from build123d import *

# Parameters (mm, degrees)
EXTRUDE_START                 = -32
EXTRUDE_15_DEPTH              = 64
CUT_EXTRUDE_1_DEPTH           = 100
CUT_EXTRUDE_1_DEPTH_BACK      = 100
SKETCH_2_R                    = 3.2
CUT_EXTRUDE_1_2_DEPTH         = 100
CUT_EXTRUDE_1_2_DEPTH_BACK    = 100
SKETCH_3_R                    = 3.2
CUT_EXTRUDE_M3_1_DEPTH        = 100
CUT_EXTRUDE_M3_1_DEPTH_BACK   = 100
SKETCH_4_R                    = 1.65
CUT_EXTRUDE_M3_1_2_DEPTH      = 100
CUT_EXTRUDE_M3_1_2_DEPTH_BACK = 100
SKETCH_5_R                    = 1.65
CUT_EXTRUDE_M3_DEPTH          = 12
CUT_EXTRUDE_M3_DEPTH_BACK     = 12
SKETCH_6_R                    = 1.65


with BuildPart() as part:
    # 草图1 → 四毫米底座及15度斜壁 (new body)
    with BuildSketch(Plane.XY.offset(EXTRUDE_START)):
        Polygon((-18, 0), (0, 0), (4.287187079, 16), (0.146082357, 16), (-3.069307952, 4), (-18, 4), align=None)
    extrude(amount=EXTRUDE_15_DEPTH)

    # 草图2 → Cut-Extrude 1 (cut, two sides: drawn at the far end of the back side and taken through both)
    with BuildSketch(Plane(origin=(0, 0, 0), x_dir=(1, 0, 0), z_dir=(0, 1, 0)).offset(-CUT_EXTRUDE_1_DEPTH_BACK)):
        with Locations((-15, 20)):
            Circle(SKETCH_2_R)
    extrude(amount=CUT_EXTRUDE_1_DEPTH + CUT_EXTRUDE_1_DEPTH_BACK, mode=Mode.SUBTRACT)

    # 草图3 → Cut-Extrude 1 2 (cut, two sides: drawn at the far end of the back side and taken through both)
    with BuildSketch(Plane(origin=(0, 0, 0), x_dir=(1, 0, 0), z_dir=(0, 1, 0)).offset(-CUT_EXTRUDE_1_2_DEPTH_BACK)):
        with Locations((-15, -20)):
            Circle(SKETCH_3_R)
    extrude(amount=CUT_EXTRUDE_1_2_DEPTH + CUT_EXTRUDE_1_2_DEPTH_BACK, mode=Mode.SUBTRACT)

    # 草图4 → Cut-Extrude M3__-1 (cut, two sides: drawn at the far end of the back side and taken through both)
    with BuildSketch(Plane(origin=(0, 0, 0), x_dir=(1, 0, 0), z_dir=(0, 1, 0)).offset(-CUT_EXTRUDE_M3_1_DEPTH_BACK)):
        with Locations(Location((-12, 28, 0), (0, 0, 270))):
            Circle(SKETCH_4_R)
    extrude(amount=CUT_EXTRUDE_M3_1_DEPTH + CUT_EXTRUDE_M3_1_DEPTH_BACK, mode=Mode.SUBTRACT)

    # 草图5 → Cut-Extrude M3__1 2 (cut, two sides: drawn at the far end of the back side and taken through both)
    with BuildSketch(Plane(origin=(0, 0, 0), x_dir=(1, 0, 0), z_dir=(0, 1, 0)).offset(-CUT_EXTRUDE_M3_1_2_DEPTH_BACK)):
        with Locations(Location((-12, -28, 0), (0, 0, 270))):
            Circle(SKETCH_5_R)
    extrude(amount=CUT_EXTRUDE_M3_1_2_DEPTH + CUT_EXTRUDE_M3_1_2_DEPTH_BACK, mode=Mode.SUBTRACT)

    # 草图6 → 长脚斜面双M3孔 (cut, two sides: drawn at the far end of the back side and taken through both)
    with BuildSketch(Plane(origin=(0, 0, 0), x_dir=(0, 0, -1), z_dir=(0.9659258262890684, -0.2588190451025208, 0)).offset(-CUT_EXTRUDE_M3_DEPTH_BACK)):
        with Locations(Location((24, 10, 0), (0, 0, 90))):
            Circle(SKETCH_6_R)
        with Locations(Location((-24, 10, 0), (0, 0, 90))):
            Circle(SKETCH_6_R)
    extrude(amount=CUT_EXTRUDE_M3_DEPTH + CUT_EXTRUDE_M3_DEPTH_BACK, mode=Mode.SUBTRACT)


solid = part.part
The model under review builds one solid part; all positions refer to its coordinate system, in mm. A direction names the side the tool comes from. Give positions to 0.01 mm unless a question says otherwise; leave off trailing zeros. Order: outer loops, then holes, each group sorted by start corner. A loop starts at its lowest first (then second) coordinate and runs counter-clockwise, first axis right, second up. Notation, with made-up numbers: M 78,-23 L 131,-23 A24 ccw 131,9 Z; hole C 29.5,82 d11. An arc over 180 degrees is marked long. Answer in a Markdown table with one row per item. Add a question column.
1. Machinability: for faces 1 (the cylindrical face through (0.574, 9.977, 25.636)), 2 (the flat face through (-10, 4, 0)), which of the approach directions +Z, -Z, +X, -X, +Y, -Y give a long, thin tool a straight path to every point of the face, cutting with its end or side? Answer none if there is none.
2. To check wall thickness, follow line 1 along Z through (x, y) = (-15, 2.85); line 2 along Y through (x, z) = (-5.25, -1); line 3 along Z through (x, y) = (-16.75, 1.5). State the ranges of each line that lie inside material, in increasing order.
3. Add section D-D on z = 20. State the section outline as (x, y) points, plus the area to 3 significant figures.
4. For pin 1 Ø12 at (x, z) = (-14, -14) entering from +Y; pin 2 Ø6 at (x, z) = (-15, 20) entering from +Y; pin 3 Ø1.5 at (y, z) = (2.5, 22) entering from +X; pin 4 Ø1 at (y, z) = (9, -6.5) entering from -X, all flat-tipped, find the tip position at first contact; note any pin that passes through.
5. Add section C-C on y = 2. State the section outline as (x, z) points.
6. Add section A-A on x = -15. State the section outline as (y, z) points, plus the area to 3 significant figures.
7. Add section B-B on z = -28. State the section outline as (x, y) points, plus the area to 3 significant figures.
8. Mouldability with a two-part tool opening along Z and no side actions: class faces 3 (the flat face through (-9, 0, 0)), 4 (the flat face through (-5, 3, -32)), 5 (the cylindrical face through (-11.8, 2, -19.9)) as released by +Z, released by -Z, zero draft, split by the parting line, or undercut.
The answers:
| question | item | result |
|---|---|---|
| 1 | face 1 | none |
| 1 | face 2 | +Z, -Z, -X, +Y |
| 2 | line 1 | -32 to -23.2, -16.8 to 16.8, 23.2 to 32 |
| 2 | line 2 | 0 to 4 |
| 2 | line 3 | -32 to -22.68, -17.32 to 17.32, 22.68 to 32 |
| 3 | outline | M -11.8,0 L 0,0 L 4.29,16 L 0.15,16 L -3.07,4 L -11.8,4 Z |
| 3 | area | 99.0 mm2 |
| 4 | pin 1 | y = 4 |
| 4 | pin 2 | through |
| 4 | pin 3 | x = 0.87 |
| 4 | pin 4 | x = -1.86 |
| 5 | outline | M -18,-32 L 0.54,-32 L 0.54,32 L -18,32 L -18,21.11 A3.2 cw long -18,18.89 L -18,-18.89 A3.2 cw long -18,-21.11 Z; hole C -12,-28 d3.3; hole C -12,28 d3.3 |
| 6 | outline | M 0,-32 L 4,-32 L 4,-23.2 L 0,-23.2 Z; M 0,-16.8 L 4,-16.8 L 4,16.8 L 0,16.8 Z; M 0,23.2 L 4,23.2 L 4,32 L 0,32 Z |
| 6 | area | 205 mm2 |
| 7 | outline | M -18,0 L -13.65,0 L -13.65,4 L -18,4 Z; M -10.35,0 L 0,0 L 4.29,16 L 0.15,16 L -3.07,4 L -10.35,4 Z |
| 7 | area | 111 mm2 |
| 8 | face 3 | zero draft |
| 8 | face 4 | released by -Z |
| 8 | face 5 | undercut |
